The drawing under review shows one solid part. Ordinate dimensions are in mm from its lowest x, y, z. A direction names the side the tool comes from. Round coordinates to 2 decimals unless told otherwise and drop trailing zeros. Write each loop counter-clockwise with the first axis right and the second up, starting at its lowest first coordinate (ties: lowest second). Pieces come first, ordered by that corner, then holes. Notation, with made-up numbers: (32, 37) - (43, 37) arc R33 ccw to (43, 73) - close; hole circle Ø10 at (26.5, 85.5). An arc over 180 degrees is marked (long way). Answer in a Markdown table with one row per item. Add a question column.
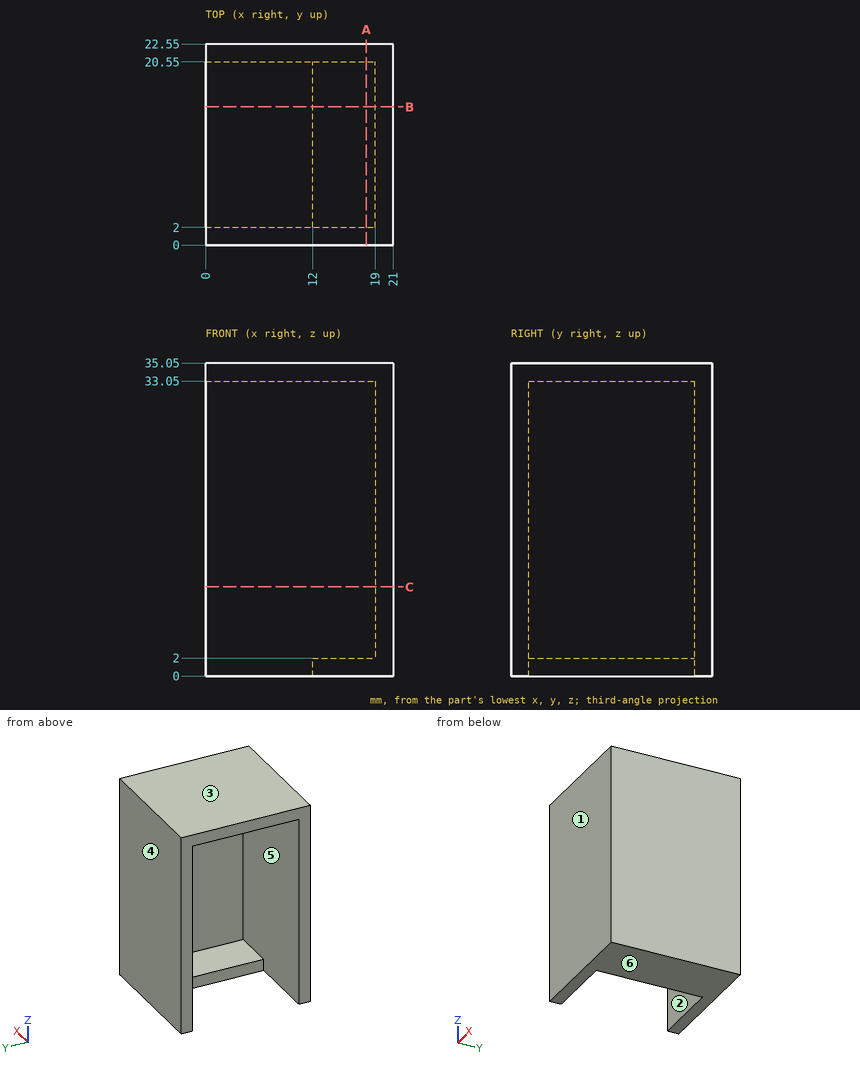
Q1. Insertion check: pin 1 Ø2 at (x, y) = (5, 13) entering from -Z; pin 2 Ø12 at (y, z) = (9, 18) entering from -X; pin 3 Ø0.6 at (y, z) = (13, 1) entering from -X. Each pin has a flat end and moves straight along its axis. Give the tip position at first contact, or say it passes through.
Q2. Add section A-A on x = 18. State the section outline as (y, z) points.
Q3. Tool access review of the marked faces 1 and 2: name each direction out of +Z, -Z, +X, -X, +Y, -Y from which nothing blocks a thin tool from reaching the whole face with its end or side.
Q4. Add section C-C on z = 10. State the section outline as (x, y) points.
Q5. Draft analysis for pull direction Z (two halves, no side actions). For the marked faces 3, 4, 5 and 6, state which applies: released by +Z, released by -Z, zero draft, split by the parting line, or undercut.
Q6. Add section B-B on y = 15.5. State the section outline as (x, z) points.
Q7. To check wall thickness, follow probe 1 along Z at (x, y) = (14.5, 7.75); probe 2 along Y at (x, z) = (13.75, 6); probe 3 along X at (y, z) = (6.25, 21). State the ranges of each line that lie inside material, in increasing order.
Answer sheet:
| question | item | result |
|---|---|---|
| 1 | pin 1 | stops at z = 33.05 |
| 1 | pin 2 | stops at x = 19 |
| 1 | pin 3 | stops at x = 12 |
| 2 | outline | (0, 0) - (22.55, 0) - (22.55, 35.05) - (0, 35.05) - close; hole (2, 2) - (20.55, 2) - (20.55, 33.05) - (2, 33.05) - close |
| 3 | face 1 | +Z, -Z, +X, -X, -Y |
| 3 | face 2 | -X |
| 4 | outline | (0, 0) - (21, 0) - (21, 22.55) - (0, 22.55) - (0, 20.55) - (19, 20.55) - (19, 2) - (0, 2) - close |
| 5 | face 3 | released by +Z |
| 5 | face 4 | zero draft |
| 5 | face 5 | undercut |
| 5 | face 6 | released by -Z |
| 6 | outline | (0, 33.05) - (19, 33.05) - (19, 2) - (12, 2) - (12, 0) - (21, 0) - (21, 35.05) - (0, 35.05) - close |
| 7 | probe 1 | z = 0 to 2, 33.05 to 35.05 |
| 7 | probe 2 | y = 0 to 2, 20.55 to 22.55 |
| 7 | probe 3 | x = 19 to 21 |
